For this review, take the finished solid that the model builds, in its own axes (mm). A direction names the side the tool comes from. Coordinates: 2 decimals unless noted, no trailing zeros. Loops run counter-clockwise (first coordinate to the right, second up) from the corner with the lowest first, then second, coordinate; pieces in that order, holes last. Notation, with made-up numbers: (-34.5, 21) - (-26.5, 21) arc R26 ccw to (-26.5, 57) - close; hole circle Ø9 at (17.5, 53). An arc over 180 degrees is marked (long way). Answer as a JSON object with one key per item and string values. Group by question number.
Item 1: We need section B-B (z = 4.1). Give the boundary of the cut face in (x, y) (3 decimals), then the cut area to 3 significant figures.
Item 2: Tool access review of faces 4 (the cylindrical face through (3.77, -131.736, 2.958)), 5 (the cylindrical face through (4.27, -158.89, 4.52)), 6 (the flat face through (4, 27, 3)): name each direction out of +Z, -Z, +X, -X, +Y, -Y from which nothing blocks a thin tool from reaching the whole face with its end or side.
Item 3: Clearance check with flat-ended pins moving along their axes: pin 1 (2 mm diameter, centred on x = 3.5, z = 5, fed in from +Y); pin 2 (3 mm diameter, centred on x = 11.5, z = 2, fed in from +Y); pin 3 (3 mm diameter, centred on x = 10, z = 2, fed in from +Y); pin 4 (16 mm diameter, centred on x = 3.04, y = -147.81, fed in from -Z). State where each tip first meets the part, or that it passes through.
Item 4: Mouldability with a two-part tool opening along Y and no side actions: class faces 1 (the cylindrical face through (-1.08, -80.73, 2.96)), 2 (the flat face through (17.891, -74, 3)), 3 (the cylindrical face through (4.27, 41.11, 1.48)) as released by +Y, released by -Y, zero draft, split by the parting line, or undercut.
Item 5: We need section A-A (y = -111.5). Give the boundary of the cut face in (x, z), then the cut area to 3 significant figures.
Item 6: We need section D-D (y = -167.5). Give the boundary of the cut face in (x, z), then the cut area to 3 significant figures.
Item 7: To check wall thickness, follow line 1 (X direction, y = -45.5, z = 4.3); line 2 (Y direction, x = -3.5, z = 2.55); line 3 (X direction, y = -72, z = 0.35). State the ranges of each line that lie inside material, in increasing order.
Item 8: We need section C-C (x = -1.75). Give the boundary of the cut face in (y, z), then the cut area to 3 significant figures.
from build123d import *

# Parameters (mm, degrees)
ESQUISSE1_W             = 27.85
ESQUISSE1_H             = 200
BOSS_EXTRU_1_DEPTH      = 6
ESQUISSE2_R             = 13.925
ENL_V_MAT_EXTRU_1_DEPTH = 3
ESQUISSE3_R             = 2.925
ENL_V_MAT_EXTRU_2_DEPTH = 3
ESQUISSE5_R             = 13.925
ENL_V_MAT_EXTRU_3_DEPTH = 3
ESQUISSE6_R             = 8.925
ESQUISSE6_W             = 17.85
ESQUISSE6_H             = 25
ENL_V_MAT_EXTRU_4_DEPTH = 10


with BuildPart() as part:
    # Esquisse1 → Boss.-Extru.1 (new body)
    with BuildSketch(Plane.XY):
        with Locations((3.966452722, -72.813095238)):
            Rectangle(ESQUISSE1_W, ESQUISSE1_H)
        with BuildLine():
            Line((-9.958547278, -172.813095238), (17.891452722, -172.813095238))
            ThreePointArc((17.891452722, -172.813095238), (3.966452722, -186.738095238), (-9.958547278, -172.813095238))
        make_face()
        with BuildLine():
            Line((-9.958547278, 27.186904762), (17.891452722, 27.186904762))
            ThreePointArc((17.891452722, 27.186904762), (3.966452722, 41.111904762), (-9.958547278, 27.186904762))
        make_face()
    extrude(amount=BOSS_EXTRU_1_DEPTH)

    # Esquisse2 → Enlèv. mat.-Extru.1 (cut)
    with BuildSketch(Plane.XY.offset(6)):
        with Locations((3.966452722, -172.813095238)):
            Circle(ESQUISSE2_R)
    extrude(amount=-ENL_V_MAT_EXTRU_1_DEPTH, mode=Mode.SUBTRACT)

    # Esquisse3 → Enlèv. mat.-Extru.2 (cut)
    with BuildSketch(Plane.XY.offset(3)):
        with Locations((3.966452722, -172.813095238)):
            Circle(ESQUISSE3_R)
    extrude(amount=-ENL_V_MAT_EXTRU_2_DEPTH, mode=Mode.SUBTRACT)

    # Esquisse5 → Enlèv. mat.-Extru.3 (cut)
    with BuildSketch(Plane.XY.offset(6)):
        with Locations((3.966452722, 27.186904762)):
            Circle(ESQUISSE5_R)
    extrude(amount=-ENL_V_MAT_EXTRU_3_DEPTH, mode=Mode.SUBTRACT)

    # Esquisse6 → Enlèv. mat.-Extru.4 (cut)
    with BuildSketch(Plane(origin=(0, 0, 0), x_dir=(-1, 0, 0), z_dir=(0, 0, -1))):
        with Locations((-3.040571359, 2.186904762)):
            Circle(ESQUISSE6_R)
        with BuildLine():
            ThreePointArc((-12.891452722, -22.813095238), (-3.966452722, -13.888095238), (4.958547278, -22.813095238))
            Line((4.958547278, -22.813095238), (-12.891452722, -22.813095238))
        make_face()
        with Locations((-3.966452722, -35.313095238)):
            Rectangle(ESQUISSE6_W, ESQUISSE6_H)
        with BuildLine():
            ThreePointArc((4.958547278, -47.813095238), (-3.966452722, -56.738095238), (-12.891452722, -47.813095238))
            Line((-12.891452722, -47.813095238), (4.958547278, -47.813095238))
        make_face()
        with Locations((-3.040571359, -72.813095238)):
            Circle(ESQUISSE6_R)
        with Locations((-3.966452722, -110.313095238)):
            Rectangle(ESQUISSE6_W, ESQUISSE6_H)
        with BuildLine():
            ThreePointArc((-12.891452722, -97.813095238), (-3.966452722, -88.888095238), (4.958547278, -97.813095238))
            Line((4.958547278, -97.813095238), (-12.891452722, -97.813095238))
        make_face()
        with BuildLine():
            ThreePointArc((4.958547278, -122.813095238), (-3.966452722, -131.738095238), (-12.891452722, -122.813095238))
            Line((-12.891452722, -122.813095238), (4.958547278, -122.813095238))
        make_face()
        with Locations((-3.040571359, -147.813095238)):
            Circle(ESQUISSE6_R)
    extrude(amount=-ENL_V_MAT_EXTRU_4_DEPTH, mode=Mode.SUBTRACT)


solid = part.part
Check sheet entries:
{
 "1": {"outline": "(-9.959, -172.813) arc R13.925 cw to (17.891, -172.813) - (17.891, 27.187) arc R13.925 cw to (-9.959, 27.187) - close; hole circle Ø17.85 at (3.041, -147.813); hole circle Ø17.85 at (3.041, -72.813); hole circle Ø17.85 at (3.041, 2.187); hole (-4.959, -122.813) arc R8.925 ccw to (12.891, -122.813) - (12.891, -97.813) arc R8.925 ccw to (-4.959, -97.813) - close; hole (-4.959, -47.813) arc R8.925 ccw to (12.891, -47.813) - (12.891, -22.813) arc R8.925 ccw to (-4.959, -22.813) - close", "area": "2,820 mm2"},
 "2": {"face 4": "+Z, -Z", "face 5": "+Z, -Y", "face 6": "+Z, +Y"},
 "3": {"pin 1": "stops at y = 13.34", "pin 2": "stops at y = 39.74", "pin 3": "stops at y = 40.35", "pin 4": "passes through"},
 "4": {"face 1": "undercut", "face 2": "zero draft", "face 3": "released by +Y"},
 "5": {"outline": "(-9.96, 0) - (-4.96, 0) - (-4.96, 6) - (-9.96, 6) - close; (12.89, 0) - (17.89, 0) - (17.89, 6) - (12.89, 6) - close", "area": "60.0 mm2"},
 "6": {"outline": "(-9.96, 0) - (17.89, 0) - (17.89, 6) - (16.84, 6) - (16.84, 3) - (-8.91, 3) - (-8.91, 6) - (-9.96, 6) - close", "area": "89.9 mm2"},
 "7": {"line 1": "x = -9.96 to -4.96, 12.89 to 17.89", "line 2": "y = -184.57 to -153.89, -141.74 to -127.7, -92.92 to -78.89, -66.74 to -52.7, -17.92 to -3.89, 8.26 to 38.94", "line 3": "x = -9.96 to -5.85, 11.93 to 17.89"},
 "8": {"outline": "(-185.51, 0) - (-155.34, 0) - (-155.34, 6) - (-160.12, 6) - (-160.12, 3) - (-185.51, 3) - close; (-140.28, 0) - (-129.67, 0) - (-129.67, 6) - (-140.28, 6) - close; (-90.96, 0) - (-80.34, 0) - (-80.34, 6) - (-90.96, 6) - close; (-65.28, 0) - (-54.67, 0) - (-54.67, 6) - (-65.28, 6) - close; (-15.96, 0) - (-5.34, 0) - (-5.34, 6) - (-15.96, 6) - close; (9.72, 0) - (39.88, 0) - (39.88, 3) - (14.49, 3) - (14.49, 6) - (9.72, 6) - close", "area": "464 mm2"}
}
